```python
from build123d import *

# Parameters (mm, degrees)
CROQUIS1_W              = 45
CROQUIS1_H              = 45
SALIENTE_EXTRUIR1_DEPTH = 500
CROQUIS2_W              = 41
CROQUIS2_H              = 41
CORTAR_EXTRUIR1_DEPTH   = 505.03372903
CROQUIS3_R              = 7
CORTAR_EXTRUIR2_DEPTH   = 505.03372903


with BuildPart() as part:
    # Croquis1 → Saliente-Extruir1 (new body)
    with BuildSketch(Plane(origin=(0, 0, 0), x_dir=(1, 0, 0), z_dir=(0, 1, 0))):
        with Locations((22.5, 22.5)):
            Rectangle(CROQUIS1_W, CROQUIS1_H)
    extrude(amount=SALIENTE_EXTRUIR1_DEPTH)

    # Croquis2 → Cortar-Extruir1 (cut, through all)
    with BuildSketch(Plane(origin=(0, 500, 0), x_dir=(1, 0, 0), z_dir=(0, 1, 0))):
        with Locations((22.5, 22.5)):
            Rectangle(CROQUIS2_W, CROQUIS2_H)
    extrude(amount=-CORTAR_EXTRUIR1_DEPTH, mode=Mode.SUBTRACT)

    # Croquis3 → Cortar-Extruir2 (cut, through all)
    with BuildSketch(Plane(origin=(45, 0, 0), x_dir=(0, 0, -1), z_dir=(1, 0, 0))):
        with Locations((22.5, 479)):
            Circle(CROQUIS3_R)
        with Locations((22.5, 21)):
            Circle(CROQUIS3_R)
    extrude(amount=-CORTAR_EXTRUIR2_DEPTH, mode=Mode.SUBTRACT)


solid = part.part
```
Design review of the part built by this model. Coordinates are the model's own, in mm. A direction names the side the tool comes from. Give positions to 0.01 mm unless a question says otherwise; leave off trailing zeros. Order: outer loops, then holes, each group sorted by start corner. A loop starts at its lowest first (then second) coordinate and runs counter-clockwise, first axis right, second up. Notation, with made-up numbers: M 25.25,-6 L 57.25,-6 A29 ccw 57.25,18 Z; hole C 65.5,57 d2. An arc over 180 degrees is marked long. One line per question, with ' | ' between items. Start each with the question number.
Q1. For L1, parallel to Y at x = 1.6, z = -22.5; L2, parallel to X at y = 427.5, z = -39; L3, parallel to Z at x = 34, y = 23, list the stretches that pass through material, from the lowest coordinate up. Write a range as [from, to].
Q2. The part is to be moulded in two halves that separate along X. For faces 1 (the face through (1.014, 14.166, -20.983)), 2 (the face through (22, 254, -2)), 3 (the face through (0, 246, -22)), say which applies: +X half, -X half, draft (parallel to the pull), parting line (faces both ways), or undercut.
Q3. For pin 1 Ø12.5 at (y, z) = (479, -22.5) entering from -X, flat-tipped, find the tip position at first contact; note if it passes through.
Q4. We need section C-C (x = 30.5). Write out the cut boundary in (y, z).
Q5. Machinability: for faces 4 (the face through (21, 0, -1)), 5 (the face through (22, 254, -43)), which of the approach directions +Z, -Z, +X, -X, +Y, -Y give a long, thin tool a straight path to every point of the face, cutting with its end or side? Answer none if there is none.
Q6. We need section D-D (y = 314). Write out the cut boundary in (x, z), plus the area to 3 significant figures.
Q7. We need section A-A (y = 479). Write out the cut boundary in (x, z), plus the area to 3 significant figures.
Q8. We need section B-B (z = -38). Write out the cut boundary in (x, y).
Returned:
1) L1: [0, 14], [28, 472], [486, 500] | L2: [0, 2], [43, 45] | L3: [-45, -43], [-2, 0]
2) face 1: draft | face 2: undercut | face 3: -X half
3) pin 1: through
4) outline: M 0,-45 L 500,-45 L 500,-43 L 0,-43 Z; M 0,-2 L 500,-2 L 500,0 L 0,0 Z
5) face 4: +Z, -Z, +X, -X, -Y | face 5: +Y, -Y
6) outline: M 0,-45 L 45,-45 L 45,0 L 0,0 Z; hole M 2,-43 L 43,-43 L 43,-2 L 2,-2 Z | area: 344 mm2
7) outline: M 0,-45 L 45,-45 L 45,-29.5 L 43,-29.5 L 43,-43 L 2,-43 L 2,-29.5 L 0,-29.5 Z; M 0,-15.5 L 2,-15.5 L 2,-2 L 43,-2 L 43,-15.5 L 45,-15.5 L 45,0 L 0,0 Z | area: 288 mm2
8) outline: M 0,0 L 2,0 L 2,500 L 0,500 Z; M 43,0 L 45,0 L 45,500 L 43,500 Z
